```python
from build123d import *

# Parameters (mm, degrees)
SKETCH006_W     = 70
SKETCH006_H     = 45
PAD004_DEPTH    = 25
POCKET002_DEPTH = 23.5
SKETCH008_R     = 2.5
SKETCH008_R_2   = 0.75
PAD005_DEPTH    = 6.5
SKETCH009_R     = 7.85
POCKET003_DEPTH = 5
SKETCH010_R     = 4
SKETCH010_R_2   = 2
POCKET004_DEPTH = 5
PAD006_DEPTH    = 1.5
FILLET_R        = 2
SKETCH012_R     = 0.75
POCKET005_DEPTH = 15


with BuildPart() as part:
    # Sketch006 (on Face1 of ReferencePocket) → Pad004 (new body)
    with BuildSketch(Plane(origin=(0, 0, 0), x_dir=(1, 0, 0), z_dir=(0, 0, -1))):
        Rectangle(SKETCH006_W, SKETCH006_H)
    extrude(amount=-PAD004_DEPTH)

    # Sketch007 (on Face6 of Pad004) → Pocket002 (cut)
    with BuildSketch(Plane.XY.offset(25)):
        Polygon((-33.5, -15.4644660941), (-33.5, 15.4644660941), (-27.9644660941, 21), (27.9644660941, 21), (33.5, 15.4644660941), (33.5, -15.4644660941), (27.9644660941, -21), (-27.9644660941, -21), align=None)
    extrude(amount=-POCKET002_DEPTH, mode=Mode.SUBTRACT)

    # Sketch008 (on Face1 of ReferencePocket) → Pad005 (join)
    with BuildSketch(Plane(origin=(0, 0, 0), x_dir=(1, 0, 0), z_dir=(0, 0, -1))):
        with Locations((-27, 6.5)):
            Circle(SKETCH008_R)
        with Locations((-27, 6.5)):
            Circle(SKETCH008_R_2, mode=Mode.SUBTRACT)
        with Locations((16, 6.5)):
            Circle(SKETCH008_R)
        with Locations((16, 6.5)):
            Circle(SKETCH008_R_2, mode=Mode.SUBTRACT)
        with Locations((16, -14.5)):
            Circle(SKETCH008_R)
        with Locations((16, -14.5)):
            Circle(SKETCH008_R_2, mode=Mode.SUBTRACT)
        with Locations((-27, -14.5)):
            Circle(SKETCH008_R)
        with Locations((-27, -14.5)):
            Circle(SKETCH008_R_2, mode=Mode.SUBTRACT)
    extrude(amount=-PAD005_DEPTH)

    # Sketch009 (on Face14 of Pad005) → Pocket003 (cut)
    with BuildSketch(Plane(origin=(33.5, 0, 0), x_dir=(0, -1, 0), z_dir=(-1, 0, 0))):
        with Locations((0, 13.25)):
            Circle(SKETCH009_R)
    extrude(amount=-POCKET003_DEPTH, mode=Mode.SUBTRACT)

    # Sketch010 (on Face1 of Pocket003) → Pocket004 (cut)
    with BuildSketch(Plane.XZ.offset(22.5)):
        with Locations((-17.5, 12.5)):
            Circle(SKETCH010_R)
        with Locations((0, 12.5)):
            Circle(SKETCH010_R_2)
        with Locations((25, 12.5)):
            Circle(SKETCH010_R_2)
        Polygon((2.5, 18.5), (22.5, 18.5), (20.5, 6.5), (4.5, 6.5), align=None)
    extrude(amount=-POCKET004_DEPTH, mode=Mode.SUBTRACT)

    # Sketch011 (on Face1 of Pocket004) → Pad006 (join)
    with BuildSketch(Plane.XZ.offset(22.5)):
        with BuildLine():
            ThreePointArc((22.3059335071, 17.3356010429), (22.0825595608, 18.1463748961), (21.3195396089, 18.5))
            Line((21.3195396089, 18.5), (22.5, 18.5))
            Line((22.5, 18.5), (22.3059335071, 17.3356010429))
        make_face()
        with BuildLine():
            ThreePointArc((3.6804604217, 18.5), (2.9174404392, 18.1463748961), (2.6940664979, 17.3356010127))
            Line((2.5, 18.5), (2.6940664979, 17.3356010127))
            Line((3.6804604217, 18.5), (2.5, 18.5))
        make_face()
        with BuildLine():
            ThreePointArc((4.3607346062, 7.3355923631), (4.7007521923, 6.7369800175), (5.3471183194, 6.5))
            Line((4.5, 6.5), (5.3471183194, 6.5))
            Line((4.3607346062, 7.3355923631), (4.5, 6.5))
        make_face()
        with BuildLine():
            ThreePointArc((19.6528729116, 6.5), (20.2992478077, 6.7369800175), (20.6392668354, 7.3356010127))
            Line((20.6392668354, 7.3356010127), (20.5, 6.5))
            Line((20.5, 6.5), (19.6528729116, 6.5))
        make_face()
    extrude(amount=-PAD006_DEPTH)

    # Fillet
    fillet_edges = [part.edges().sort_by_distance(p)[0] for p in [
        (35, -22.5, 12.5),
        (-35, -22.5, 12.5),
        (35, 22.5, 12.5),
        (-35, 22.5, 12.5),
    ]]
    fillet(fillet_edges, radius=FILLET_R)

    # Sketch012 (on Face5 of Fillet) → Pocket005 (cut)
    with BuildSketch(Plane.XY.offset(25)):
        with Locations((-32.3661165235, 19.8661165235)):
            Circle(SKETCH012_R)
        with Locations((32.3661165235, 19.8661165235)):
            Circle(SKETCH012_R)
        with Locations((32.3661165235, -19.8661165235)):
            Circle(SKETCH012_R)
        with Locations((-32.3661165235, -19.8661165235)):
            Circle(SKETCH012_R)
    extrude(amount=-POCKET005_DEPTH, mode=Mode.SUBTRACT)


solid = part.part
```
Work out the finished part from the listing and answer in its coordinate system (mm). A direction names the side the tool comes from. Give positions to 0.01 mm unless a question says otherwise; leave off trailing zeros. Loops run counter-clockwise (first coordinate to the right, second up) from the corner with the lowest first, then second, coordinate; pieces in that order, holes last. Notation, with made-up numbers: M 77,77.25 L 81,77.25 A25 ccw 81,107.25 Z; hole C -38,-2 d5. An arc over 180 degrees is marked long. One line per item, written item: value. Start each with the question number.
1. Determine the mould class of faces 1 (the face through (0, -22, 25)), 2 (the face through (16, -6, 1.5)), 3 (the face through (-34.43, 21.9, 12.68)), 4 (the face through (-32.02, -20.53, 17.6)) for opening direction Y: released by +Y, released by -Y, zero draft, split by the parting line, or undercut.
2. Each of these flat-tipped pins is pushed along its axis until it touches: P1, Ø0.9, axis at x = -27, y = -6.5, coming from the +Z side; P2, Ø3, axis at y = -1, z = 19, coming from the +X side; P3, Ø2.5, axis at x = -26.5, y = -7.5, coming from the +Z side. Where does it stop, or does it pass through?
3. Find section D-D (y = -13.5). Give the vertices of the cut face in (x, z), and give its area (4 significant figures).
4. Which of the six approach directions +Z, -Z, +X, -X, +Y, -Y give full straight-line access (tool end or side, diameter ignored) to faces 5 (the face through (-27.595, -6.044, 3.965)), 6 (the face through (15, 15, 6.5)), 7 (the face through (3.54, -21.76, 12.27))?
5. Find section B-B (y = 0). Give the vertices of the cut face in (x, z), and give its area (3 significant figures).
6. Find section C-C (z = 15.5). State how many separate pieces and enclosed holes the cut face has, and give its area (3 significant figures).
7. Find the intervals of material crossed by probe 1 along Y at (x, z) = (16, 3.05); probe 2 along X at (y, z) = (7, 21.25); probe 3 along Y at (x, z) = (0.5, 3.5), in increasing order.
8. Find section A-A (x = 25). Give the vertices of the cut face in (y, z), and give its area (3 significant figures).
Reported:
1. face 1: zero draft
1. face 2: undercut
1. face 3: released by +Y
1. face 4: undercut
2. P1: stops at z = 1.5
2. P2: stops at x = -33.5
2. P3: stops at z = 6.5
3. outline: M -35,0 L 35,0 L 35,25 L 33.5,25 L 33.5,1.5 L -33.5,1.5 L -33.5,25 L -35,25 Z
3. area: 175.5 mm²
4. face 5: +Z
4. face 6: +Z, -Y
4. face 7: -Y
5. outline: M -35,0 L 35,0 L 35,5.4 L 33.5,5.4 L 33.5,1.5 L -33.5,1.5 L -33.5,25 L -35,25 Z; M 33.5,21.1 L 35,21.1 L 35,25 L 33.5,25 Z
5. area: 152 mm²
6. separate pieces: 3
6. enclosed holes: 4
6. area: 328 mm²
7. probe 1: y = -22.5 to -21, -9 to -7.25, -5.75 to -4, 12 to 13.75, 15.25 to 17, 21 to 22.5
7. probe 2: x = -35 to -33.5, 33.5 to 35
7. probe 3: y = -22.5 to -21, 21 to 22.5
8. outline: M -22.5,0 L 22.5,0 L 22.5,25 L 21,25 L 21,1.5 L -21,1.5 L -21,10.5 L -22.5,10.5 Z; M -22.5,14.5 L -21,14.5 L -21,25 L -22.5,25 Z
8. area: 132 mm²
